Design review of the part built by this model. Coordinates are the model's own, in mm. Face numbers are marked on the shaded views. A direction names the side the tool comes from. Round coordinates to 2 decimals unless told otherwise and drop trailing zeros. Loops run counter-clockwise (first coordinate to the right, second up) from the corner with the lowest first, then second, coordinate; pieces in that order, holes last. Notation, with made-up numbers: (-14, 77) - (-8, 77) arc R8 ccw to (-8, 86) - close; hole circle Ø5 at (49.5, -19.75). An arc over 180 degrees is marked (long way). Use one line per item in the form item = value. Start each with the question number.
(1) Machinability: for the marked faces 1 and 2, which of the approach directions +Z, -Z, +X, -X, +Y, -Y give a long, thin tool a straight path to every point of the face, cutting with its end or side? Answer none if there is none.
(2) We need section A-A, the plane y = 0. Write out the cut boundary in (x, z).
(3) For pin 1 (3 mm diameter, centred on x = -2, z = 6, fed in from +Y); pin 2 (10 mm diameter, centred on x = -19, z = 3, fed in from -Y); pin 3 (1 mm diameter, centred on x = 0, z = 3, fed in from -Y), all flat-tipped, find the tip position at first contact; note any pin that passes through.
(4) Wall thickness on probe 1 along X at (y, z) = (5.5, -6.25); probe 2 along Y at (x, z) = (-0.5, -4.25); probe 3 along X at (y, z) = (4.5, -1.5): over which ranges is each line inside the solid? List them lowest first. Write a range as [from, to].
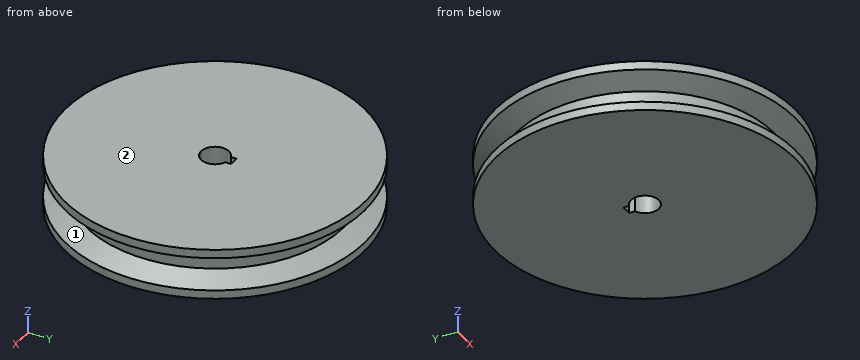
from build123d import *

# Parameters (mm, degrees)
PAD_DEPTH = 8.5


with BuildPart() as part:
    # Sketch → Pad (new body, symmetric)
    with BuildSketch(Plane.XY):
        with BuildLine():
            ThreePointArc((0, -4.65), (4.573728, -0.838758), (1.65, 4.347413))
            Line((1.65, 6.25), (1.65, 4.347413))
            Line((0, 6.25), (1.65, 6.25))
            Line((0, 50), (0, 6.25))
            ThreePointArc((0, -50), (50, 0), (0, 50))
            Line((0, -4.65), (0, -50))
        make_face()
    pad = extrude(amount=PAD_DEPTH, both=True)

    # Mirrored: Pad across Sketch V_Axis
    add(pad.mirror(Plane(origin=(0, 0, 0), x_dir=(0, 0, 1), z_dir=(1, 0, 0))))

    # Sketch001 → Groove (revolve, cut)
    with BuildSketch(Plane.YZ):
        Polygon((50, 0), (50, 5.6), (43, 2.6), (43, 0), align=None)
    groove = revolve(axis=Axis((0, 0, 0), (0, 0, 1)), mode=Mode.SUBTRACT)

    # Mirrored001: Groove across Sketch001 H_Axis
    add(groove.mirror(Plane.XY), mode=Mode.SUBTRACT)


solid = part.part
Data:
q1.face_1 = none
q1.face_2 = +Z, +X, -X, +Y, -Y
q2.outline = (-50, -8.5) - (-4.65, -8.5) - (-4.65, 8.5) - (-50, 8.5) - (-50, 5.6) - (-43, 2.6) - (-43, -2.6) - (-50, -5.6) - close; (4.65, -8.5) - (50, -8.5) - (50, -5.6) - (43, -2.6) - (43, 2.6) - (50, 5.6) - (50, 8.5) - (4.65, 8.5) - close
q3.pin_1 = 50
q3.pin_2 = -47.78
q3.pin_3 = -45.1
q4.probe_1 = [-49.7, -1.65], [1.65, 49.7]
q4.probe_2 = [-46.85, -4.62], [6.25, 46.85]
q4.probe_3 = [-42.76, -1.65], [1.65, 42.76]
